Build history of the part. All positions in model axes, mm. Coordinates: 2 decimals unless noted, no trailing zeros. Write each loop counter-clockwise with the first axis right and the second up, starting at its lowest first coordinate (ties: lowest second). Pieces come first, ordered by that corner, then holes.
```python
from build123d import *

# Parameters (mm, degrees)
F0_W     = 170
F0_H     = 90
F1_DEPTH = 2.54
F2_R     = 12.5
F3_DEPTH = 2.541
F4_R     = 2.5
F5_DEPTH = 2.541


with BuildPart() as f1:
    # F0 (on Top) → F1 (new body)
    with BuildSketch(Plane.XY):
        Rectangle(F0_W, F0_H)
    extrude(amount=F1_DEPTH)

    # F2 (on face) → F3 (cut, through all)
    with BuildSketch(Plane.XY.offset(2.54)):
        Circle(F2_R)
    extrude(amount=-F3_DEPTH, mode=Mode.SUBTRACT)

    # F4 (on face) → F5 (cut, through all)
    with BuildSketch(Plane.XY.offset(2.54)):
        with Locations((-72.5, 32.5)):
            Circle(F4_R)
        with Locations((72.5, 32.5)):
            Circle(F4_R)
        with Locations((72.5, -32.5)):
            Circle(F4_R)
        with Locations((-72.5, -32.5)):
            Circle(F4_R)
    extrude(amount=-F5_DEPTH, mode=Mode.SUBTRACT)


solid = f1.part
```
1. Probe line 1 along Y through (x, z) = (-72.5, 0.9); line 2 along X through (y, z) = (0.5, 1.35); line 3 along X through (y, z) = (-31, 1.4). List the from-to ranges inside material, lowest first.
Computed values:
line 1: y = -45 to -35, -30 to 30, 35 to 45
line 2: x = -85 to -12.49, 12.49 to 85
line 3: x = -85 to -74.5, -70.5 to 70.5, 74.5 to 85
2. Flat gauge pin, fed straight in: pin 1 (6 mm diameter, centred on x = -72.5, y = -32.5, fed in from +Z). Where does the tip first touch, or does it go through?
Computed values:
pin 1: stops at z = 2.54
3. Mould opens along Y. For faces 1 (the face through (-20, 1, 2.54)), 2 (the face through (-74.34, -30.81, 1.29)) say: +Y half, -Y half, draft (parallel to the pull), parting line (faces both ways), or undercut.
Computed values:
face 1: draft
face 2: undercut
4. Saw through at A-A on x = 0. List the corners of the cut face in (y, z).
Computed values:
outline: (-45, 0) - (-12.5, 0) - (-12.5, 2.54) - (-45, 2.54) - close; (12.5, 0) - (45, 0) - (45, 2.54) - (12.5, 2.54) - close
5. Saw through at B-B on y = -32.5. List the corners of the cut face in (x, z), plus the area to 3 significant figures.
Computed values:
outline: (-85, 0) - (-75, 0) - (-75, 2.54) - (-85, 2.54) - close; (-70, 0) - (70, 0) - (70, 2.54) - (-70, 2.54) - close; (75, 0) - (85, 0) - (85, 2.54) - (75, 2.54) - close
area: 406 mm2
6. Saw through at D-D on z = 0.6. List the corners of the cut face in (x, y), plus the area to 3 significant figures.
Computed values:
outline: (-85, -45) - (85, -45) - (85, 45) - (-85, 45) - close; hole circle Ø5 at (-72.5, -32.5); hole circle Ø5 at (-72.5, 32.5); hole circle Ø25 at (0, 0); hole circle Ø5 at (72.5, -32.5); hole circle Ø5 at (72.5, 32.5)
area: 14,700 mm2
7. Saw through at C-C on x = -72.5. List the corners of the cut face in (y, z), plus the area to 3 significant figures.
Computed values:
outline: (-45, 0) - (-35, 0) - (-35, 2.54) - (-45, 2.54) - close; (-30, 0) - (30, 0) - (30, 2.54) - (-30, 2.54) - close; (35, 0) - (45, 0) - (45, 2.54) - (35, 2.54) - close
area: 203 mm2
